```python
from build123d import *

# Parameters (mm, degrees)
SKETCH1_R           = 5
BOSS_EXTRUDE1_DEPTH = 220
SKETCH4_R           = 3.2
BOSS_EXTRUDE3_DEPTH = 6
BOSS_EXTRUDE4_DEPTH = 220
SKETCH5_R           = 1.37
CUT_EXTRUDE1_DEPTH  = 7
SKETCH6_R           = 1.37
CUT_EXTRUDE2_DEPTH  = 7
SKETCH7_R           = 3.2
CUT_EXTRUDE3_DEPTH  = 6
CUT_EXTRUDE4_DEPTH  = 11.4
SKETCH10_R          = 2
CUT_EXTRUDE5_DEPTH  = 7
CUT_EXTRUDE6_DEPTH  = 11.4
SKETCH12_R          = 2
CUT_EXTRUDE7_DEPTH  = 7


with BuildPart() as part:
    # Sketch1 → Boss-Extrude1 (new body)
    with BuildSketch(Plane.XY):
        Circle(SKETCH1_R)
        with BuildLine():
            Line((-4, -3), (-7, -8.196152423))
            Line((-7, -8.196152423), (7, -8.196152423))
            Line((7, -8.196152423), (4, -3))
            ThreePointArc((4, -3), (0, 5), (-4, -3))
        make_face()
        with BuildLine():
            Line((28.8, -3), (31.8, -8.196152423))
            Line((31.8, -8.196152423), (17.8, -8.196152423))
            Line((17.8, -8.196152423), (20.8, -3))
            ThreePointArc((20.8, -3), (24.8, 5), (28.8, -3))
        make_face()
    extrude(amount=BOSS_EXTRUDE1_DEPTH)

    # Sketch4 → Boss-Extrude3 (add)
    with BuildSketch(Plane.XZ.offset(8.196152423)):
        with Locations((0, 196.8)):
            Circle(SKETCH4_R)
        with Locations((24.8, 196.8)):
            Circle(SKETCH4_R)
        with Locations((24.8, 172)):
            Circle(SKETCH4_R)
        with Locations((24.8, 147.2)):
            Circle(SKETCH4_R)
        with Locations((24.8, 122.4)):
            Circle(SKETCH4_R)
        with Locations((24.8, 97.6)):
            Circle(SKETCH4_R)
        with Locations((24.8, 72.8)):
            Circle(SKETCH4_R)
        with Locations((24.8, 48)):
            Circle(SKETCH4_R)
        with Locations((24.8, 23.2)):
            Circle(SKETCH4_R)
        with Locations((0, 172)):
            Circle(SKETCH4_R)
        with Locations((0, 147.2)):
            Circle(SKETCH4_R)
        with Locations((0, 122.4)):
            Circle(SKETCH4_R)
        with Locations((0, 97.6)):
            Circle(SKETCH4_R)
        with Locations((0, 72.8)):
            Circle(SKETCH4_R)
        with Locations((0, 48)):
            Circle(SKETCH4_R)
        with Locations((0, 23.2)):
            Circle(SKETCH4_R)
    extrude(amount=BOSS_EXTRUDE3_DEPTH)

    # Sketch3 → Boss-Extrude4 (add)
    with BuildSketch(Plane.XY.offset(220)):
        Polygon((7, -8.196152423), (17.8, -8.196152423), (18.65, -8.196152423), (18.65, -6.723909236), (6.15, -6.723909236), (6.15, -8.196152423), align=None)
    extrude(amount=-BOSS_EXTRUDE4_DEPTH)

    # Sketch5 → Cut-Extrude1 (cut)
    with BuildSketch(Plane(origin=(0, 0, 0), x_dir=(-1, 0, 0), z_dir=(0, 0, -1))):
        Circle(SKETCH5_R)
        with Locations((-24.8, 0)):
            Circle(SKETCH5_R)
    extrude(amount=-CUT_EXTRUDE1_DEPTH, mode=Mode.SUBTRACT)

    # Sketch6 → Cut-Extrude2 (cut)
    with BuildSketch(Plane.XY.offset(220)):
        Circle(SKETCH6_R)
        with Locations((24.8, 0)):
            Circle(SKETCH6_R)
    extrude(amount=-CUT_EXTRUDE2_DEPTH, mode=Mode.SUBTRACT)

    # Sketch7 → Cut-Extrude3 (cut)
    with BuildSketch(Plane.XZ.offset(14.196152423)):
        with Locations((0, 172)):
            Circle(SKETCH7_R)
        with Locations((24.8, 172)):
            Circle(SKETCH7_R)
        with Locations((24.8, 147.2)):
            Circle(SKETCH7_R)
        with Locations((24.8, 122.4)):
            Circle(SKETCH7_R)
        with Locations((24.8, 97.6)):
            Circle(SKETCH7_R)
        with Locations((24.8, 72.8)):
            Circle(SKETCH7_R)
        with Locations((24.8, 48)):
            Circle(SKETCH7_R)
        with Locations((0, 147.2)):
            Circle(SKETCH7_R)
        with Locations((0, 122.4)):
            Circle(SKETCH7_R)
        with Locations((0, 97.6)):
            Circle(SKETCH7_R)
        with Locations((0, 72.8)):
            Circle(SKETCH7_R)
        with Locations((0, 48)):
            Circle(SKETCH7_R)
    extrude(amount=-CUT_EXTRUDE3_DEPTH, mode=Mode.SUBTRACT)

    # Sketch9 → Cut-Extrude4 (cut)
    with BuildSketch(Plane(origin=(0, 0, 0), x_dir=(-1, 0, 0), z_dir=(0, 0, -1))):
        with BuildLine():
            Line((4, -3), (7, -8.196152423))
            Line((7, -8.196152423), (-31.8, -8.196152423))
            Line((-31.8, -8.196152423), (-28.8, -3))
            ThreePointArc((-28.8, -3), (-24.8, 5), (-20.8, -3))
            Line((-20.8, -3), (-18.65, -6.723909236))
            Line((-18.65, -6.723909236), (-6.15, -6.723909236))
            Line((-6.15, -6.723909236), (-4, -3))
            ThreePointArc((-4, -3), (0, 5), (4, -3))
        make_face()
    extrude(amount=-CUT_EXTRUDE4_DEPTH, mode=Mode.SUBTRACT)

    # Sketch10 → Cut-Extrude5 (cut)
    with BuildSketch(Plane(origin=(0, 0, 11.4), x_dir=(-1, 0, 0), z_dir=(0, 0, -1))):
        with Locations((-24.8, 0)):
            Circle(SKETCH10_R)
        Circle(SKETCH10_R)
    extrude(amount=-CUT_EXTRUDE5_DEPTH, mode=Mode.SUBTRACT)

    # Sketch11 → Cut-Extrude6 (cut)
    with BuildSketch(Plane.XY.offset(220)):
        with BuildLine():
            Line((20.8, -3), (18.65, -6.723909236))
            Line((18.65, -6.723909236), (6.15, -6.723909236))
            Line((6.15, -6.723909236), (4, -3))
            ThreePointArc((4, -3), (0, 5), (-4, -3))
            Line((-4, -3), (-7, -8.196152423))
            Line((-7, -8.196152423), (31.8, -8.196152423))
            Line((31.8, -8.196152423), (28.8, -3))
            ThreePointArc((28.8, -3), (24.8, 5), (20.8, -3))
        make_face()
    extrude(amount=-CUT_EXTRUDE6_DEPTH, mode=Mode.SUBTRACT)

    # Sketch12 → Cut-Extrude7 (cut)
    with BuildSketch(Plane.XY.offset(208.6)):
        Circle(SKETCH12_R)
        with Locations((24.8, 0)):
            Circle(SKETCH12_R)
    extrude(amount=-CUT_EXTRUDE7_DEPTH, mode=Mode.SUBTRACT)


solid = part.part
```
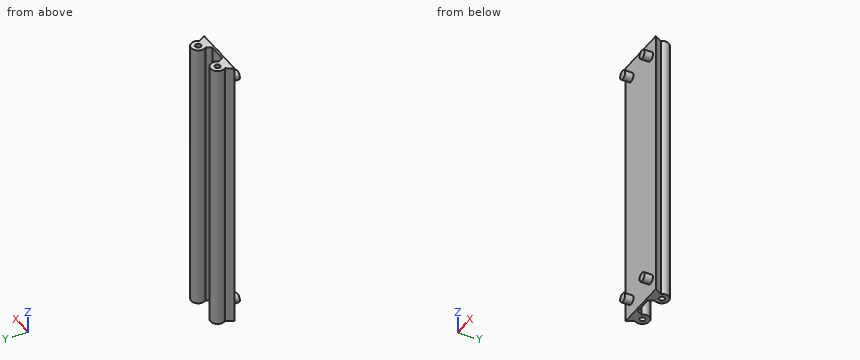
Here's how the part is built. I have some questions about the finished solid (model axes, mm). Round coordinates to 2 decimals unless told otherwise and drop trailing zeros. Order: outer loops, then holes, each group sorted by start corner. A loop starts at its lowest first (then second) coordinate and runs counter-clockwise, first axis right, second up. Notation, with made-up numbers: (21.25, -9.75) -> (59.25, -9.75) arc R22 cw to (59.25, 8.25) -> close; hole circle Ø8 at (-27.5, 9.25). An arc over 180 degrees is marked (long way). Use a Markdown table: item, result. Add a question column.
(1) I need wall thicknesses on line 1 along Z through (x, y) = (-0.5, -13); line 2 along Y through (x, z) = (12.5, 37); line 3 along X through (y, z) = (-4.25, 152). Which ranges of each line are inside material? Lowest first, please.
(2) Suppose I cut it at A-A, the plane y = 0. Please give me the cut outline in (x, z).
(3) Suppose I cut it at D-D, the plane y = -10. Please give me the cut outline in (x, z), and give its area (3 significant figures).
(4) For pin 1 Ø5 at (x, z) = (13, 109.5) entering from +Y; pin 2 Ø3 at (x, z) = (6, 172.5) entering from +Y; pin 3 Ø2.5 at (x, y) = (0, 0) entering from -Z, each with a flat end and sliding along its axis, tell me the tip position at first contact or that it passes through.
(5) Suppose I cut it at C-C, the plane x = 0. Please give me the cut outline in (y, z).
(6) Suppose I cut it at B-B, the plane z = 196.8. Please give me the cut outline in (x, y).
Verdict:
| question | item | result |
|---|---|---|
| 1 | line 1 | 20.04 to 26.36, 193.64 to 199.96 |
| 1 | line 2 | -8.2 to -6.72 |
| 1 | line 3 | -4.72 to 4.72, 20.08 to 29.52 |
| 2 | outline | (-5, 11.4) -> (-2, 11.4) -> (-2, 18.4) -> (2, 18.4) -> (2, 11.4) -> (5, 11.4) -> (5, 208.6) -> (2, 208.6) -> (2, 201.6) -> (-2, 201.6) -> (-2, 208.6) -> (-5, 208.6) -> close; (19.8, 11.4) -> (22.8, 11.4) -> (22.8, 18.4) -> (26.8, 18.4) -> (26.8, 11.4) -> (29.8, 11.4) -> (29.8, 208.6) -> (26.8, 208.6) -> (26.8, 201.6) -> (22.8, 201.6) -> (22.8, 208.6) -> (19.8, 208.6) -> close |
| 3 | outline | circle Ø6.4 at (0, 23.2); circle Ø6.4 at (0, 196.8); circle Ø6.4 at (24.8, 23.2); circle Ø6.4 at (24.8, 196.8) |
| 3 | area | 129 mm2 |
| 4 | pin 1 | y = -6.72 |
| 4 | pin 2 | y = 2.18 |
| 4 | pin 3 | z = 18.4 |
| 5 | outline | (-14.2, 20) -> (-8.2, 20) -> (-8.2, 11.4) -> (-2, 11.4) -> (-2, 18.4) -> (2, 18.4) -> (2, 11.4) -> (5, 11.4) -> (5, 208.6) -> (2, 208.6) -> (2, 201.6) -> (-2, 201.6) -> (-2, 208.6) -> (-8.2, 208.6) -> (-8.2, 200) -> (-14.2, 200) -> (-14.2, 193.6) -> (-8.2, 193.6) -> (-8.2, 26.4) -> (-14.2, 26.4) -> close |
| 6 | outline | (-7, -8.2) -> (-3.2, -8.2) -> (-3.2, -14.2) -> (3.2, -14.2) -> (3.2, -8.2) -> (21.6, -8.2) -> (21.6, -14.2) -> (28, -14.2) -> (28, -8.2) -> (31.8, -8.2) -> (28.8, -3) arc R5 ccw (long way) to (20.8, -3) -> (18.65, -6.72) -> (6.15, -6.72) -> (4, -3) arc R5 ccw (long way) to (-4, -3) -> close |
